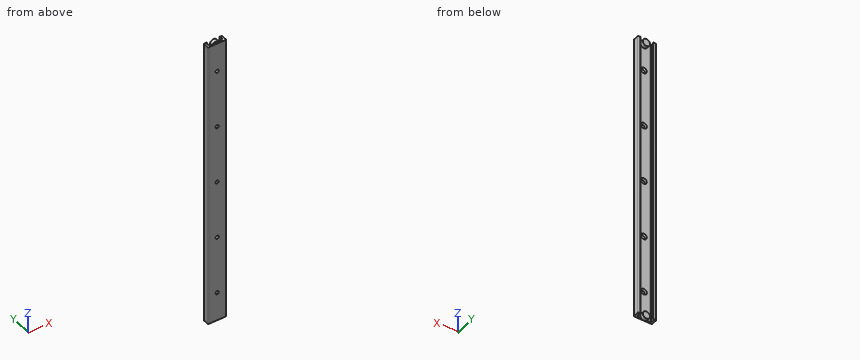
```python
from build123d import *

# Parameters (mm, degrees)
BOSS_EXTRUDE1_DEPTH = 400
SKETCH7_R           = 5
BOSS_EXTRUDE2_DEPTH = 5
SKETCH8_R           = 5
BOSS_EXTRUDE3_DEPTH = 5


with BuildPart() as part:
    # Sketch1 → Boss-Extrude1 (new body)
    with BuildSketch(Plane.XY):
        with BuildLine():
            Line((-11.5, 0), (11.5, 0))
            ThreePointArc((11.5, 0), (12.207106781, 0.292893219), (12.5, 1))
            Line((12.5, 1), (12.5, 7.5))
            ThreePointArc((12.5, 7.5), (12.207106781, 8.207106781), (11.5, 8.5))
            Line((11.5, 8.5), (9.5, 8.5))
            ThreePointArc((9.5, 8.5), (8.97237829, 8.349479447), (8.603592403, 7.943230663))
            ThreePointArc((8.603592403, 7.943230663), (9.999347871, 5.642901666), (8.5, 3.408712153))
            Line((8.5, 3.408712153), (8.5, 2.5))
            ThreePointArc((8.5, 2.5), (8.353553391, 2.146446609), (8, 2))
            Line((8, 2), (-8, 2))
            ThreePointArc((-8, 2), (-8.353553391, 2.146446609), (-8.5, 2.5))
            Line((-8.5, 2.5), (-8.5, 3.408712153))
            ThreePointArc((-8.5, 3.408712153), (-9.999347871, 5.642901666), (-8.603592403, 7.943230663))
            ThreePointArc((-8.603592403, 7.943230663), (-8.97237829, 8.349479447), (-9.5, 8.5))
            Line((-9.5, 8.5), (-11.5, 8.5))
            ThreePointArc((-11.5, 8.5), (-12.207106781, 8.207106781), (-12.5, 7.5))
            Line((-12.5, 7.5), (-12.5, 1))
            ThreePointArc((-12.5, 1), (-12.207106781, 0.292893219), (-11.5, 0))
        make_face()
    extrude(amount=BOSS_EXTRUDE1_DEPTH)

    # Sketch2 → Cut-Revolve1 (revolve, cut)
    with BuildSketch(Plane.XY.offset(40), mode=Mode.PRIVATE) as cut_revolve1_sk:
        Polygon((0, 2), (4, 2), (2.25, 0), (0, 0), align=None)
    revolve(cut_revolve1_sk.sketch.rotate(Axis((0, 0, 40), (0, 1, 0)), 270), axis=Axis((0, 0, 40), (0, 1, 0)), mode=Mode.SUBTRACT)

    # Sketch3 → Cut-Revolve2 (revolve, cut)
    with BuildSketch(Plane.XY.offset(120), mode=Mode.PRIVATE) as cut_revolve2_sk:
        Polygon((0, 2), (4, 2), (2.25, 0), (0, 0), align=None)
    revolve(cut_revolve2_sk.sketch.rotate(Axis((0, 0, 120), (0, 1, 0)), 270), axis=Axis((0, 0, 120), (0, 1, 0)), mode=Mode.SUBTRACT)

    # Sketch4 → Cut-Revolve3 (revolve, cut)
    with BuildSketch(Plane.XY.offset(200), mode=Mode.PRIVATE) as cut_revolve3_sk:
        Polygon((0, 2), (4, 2), (2.25, 0), (0, 0), align=None)
    revolve(cut_revolve3_sk.sketch.rotate(Axis((0, 0, 200), (0, 1, 0)), 270), axis=Axis((0, 0, 200), (0, 1, 0)), mode=Mode.SUBTRACT)

    # Sketch5 → Cut-Revolve4 (revolve, cut)
    with BuildSketch(Plane.XY.offset(280), mode=Mode.PRIVATE) as cut_revolve4_sk:
        Polygon((0, 2), (4, 2), (2.25, 0), (0, 0), align=None)
    revolve(cut_revolve4_sk.sketch.rotate(Axis((0, 0, 280), (0, 1, 0)), 270), axis=Axis((0, 0, 280), (0, 1, 0)), mode=Mode.SUBTRACT)

    # Sketch6 → Cut-Revolve5 (revolve, cut)
    with BuildSketch(Plane.XY.offset(360), mode=Mode.PRIVATE) as cut_revolve5_sk:
        Polygon((0, 2), (4, 2), (2.25, 0), (0, 0), align=None)
    revolve(cut_revolve5_sk.sketch.rotate(Axis((0, 0, 360), (0, 1, 0)), 270), axis=Axis((0, 0, 360), (0, 1, 0)), mode=Mode.SUBTRACT)

    # Sketch7 → Boss-Extrude2 (add)
    with BuildSketch(Plane(origin=(0, 2, 0), x_dir=(1, 0, 0), z_dir=(0, 1, 0))):
        with Locations(Location((0, -3, 0), (0, 0, 143.130102354))):
            Circle(SKETCH7_R)
    extrude(amount=BOSS_EXTRUDE2_DEPTH)

    # Sketch8 → Boss-Extrude3 (add)
    with BuildSketch(Plane(origin=(0, 2, 0), x_dir=(1, 0, 0), z_dir=(0, 1, 0))):
        with Locations(Location((0, -397, 0), (0, 0, 216.869897646))):
            Circle(SKETCH8_R)
    extrude(amount=BOSS_EXTRUDE3_DEPTH)


solid = part.part
```
Can you work these out from the model? Positions are in its coordinate system, mm. Coordinates: 2 decimals unless noted, no trailing zeros. Loops run counter-clockwise (first coordinate to the right, second up) from the corner with the lowest first, then second, coordinate; pieces in that order, holes last. Notation, with made-up numbers: (-13.75, -23) - (28.25, -23) arc R29 ccw to (28.25, 15) - close; hole circle Ø10 at (80, 33). An arc over 180 degrees is marked (long way). Use a Markdown table: item, result.
Item 1: I want a section at B-B on z = 220. Please give me the cut outline in (x, y).
Numbers:
| item | result |
|---|---|
| outline | (-12.5, 1) arc R1 ccw to (-11.5, 0) - (11.5, 0) arc R1 ccw to (12.5, 1) - (12.5, 7.5) arc R1 ccw to (11.5, 8.5) - (9.5, 8.5) arc R1 ccw to (8.6, 7.94) arc R2.5 cw to (8.5, 3.41) - (8.5, 2.5) arc R0.5 cw to (8, 2) - (-8, 2) arc R0.5 cw to (-8.5, 2.5) - (-8.5, 3.41) arc R2.5 cw to (-8.6, 7.94) arc R1 ccw to (-9.5, 8.5) - (-11.5, 8.5) arc R1 ccw to (-12.5, 7.5) - close |
Item 2: Will these pins go through, and if not, where does the flat tip stop? pin 1 (1.6 mm diameter, centred on x = -1, z = 401, fed in from -Y); pin 2 (4 mm diameter, centred on x = -4, y = 3.5, fed in from +Z); pin 3 (5 mm diameter, centred on x = 0, z = 2.5, fed in from +Y).
Numbers:
| item | result |
|---|---|
| pin 1 | stops at y = 2 |
| pin 2 | stops at z = 401.58 |
| pin 3 | stops at y = 7 |
Item 3: If I drill on probe 1 along Y at (x, z) = (-1.75, 79.5); probe 2 along X at (y, z) = (6.25, 273); probe 3 along Z at (x, y) = (-2, 6.5), over which ranges is the centre line in solid material (lowest first)? Write a range as from..to.
Numbers:
| item | result |
|---|---|
| probe 1 | y = 0..2 |
| probe 2 | x = -12.5..-9.94, 9.94..12.5 |
| probe 3 | z = -1.58..7.58, 392.42..401.58 |
Item 4: I want a section at A-A on x = 0. Give the number of separate pieces and of enclosed holes in the cut face, and give its area (4 significant figures).
Numbers:
| item | result |
|---|---|
| separate pieces | 6 |
| enclosed holes | 0 |
| area | 837.5 mm2 |
